from build123d import *

# Parameters (mm, degrees)
SKETCH2_W           = 1250
SKETCH2_H           = 250
BOSS_EXTRUDE1_DEPTH = 10
SKETCH3_W           = 25
SKETCH3_H           = 250
BOSS_EXTRUDE2_DEPTH = 300
SKETCH4_W           = 15
SKETCH4_H           = 10
BOSS_EXTRUDE3_DEPTH = 1200
FILLET1_R           = 5
FILLET3_R           = 5


with BuildPart() as part:
    # Sketch2 → Boss-Extrude1 (new body)
    with BuildSketch(Plane(origin=(0, 0, 0), x_dir=(1, 0, 0), z_dir=(0, 1, 0))):
        with Locations((546.563322885, -102.85317352)):
            Rectangle(SKETCH2_W, SKETCH2_H)
    extrude(amount=BOSS_EXTRUDE1_DEPTH)

    # Sketch3 → Boss-Extrude2 (add)
    with BuildSketch(Plane(origin=(0, 10, 0), x_dir=(1, 0, 0), z_dir=(0, 1, 0))):
        with Locations((-65.936677115, -102.85317352)):
            Rectangle(SKETCH3_W, SKETCH3_H)
        with Locations((1159.063322885, -102.85317352)):
            Rectangle(SKETCH3_W, SKETCH3_H)
    extrude(amount=BOSS_EXTRUDE2_DEPTH)

    # Sketch4 → Boss-Extrude3 (add)
    with BuildSketch(Plane(origin=(-53.436677115, 0, 0), x_dir=(0, 0, -1), z_dir=(1, 0, 0))):
        with Locations((-170.35317352, 175)):
            Rectangle(SKETCH4_W, SKETCH4_H)
        with Locations((-35.35317352, 175)):
            Rectangle(SKETCH4_W, SKETCH4_H)
    extrude(amount=BOSS_EXTRUDE3_DEPTH)

    # Fillet1
    fillet1_edges = [part.edges().sort_by_distance(p)[0] for p in [
        (546.563322885, 170, 177.85317352),
        (546.563322885, 170, 162.85317352),
    ]]
    fillet(fillet1_edges, radius=FILLET1_R)

    # Fillet3
    fillet3_edges = [part.edges().sort_by_distance(p)[0] for p in [
        (546.563322885, 170, 42.85317352),
        (546.563322885, 170, 27.85317352),
    ]]
    fillet(fillet3_edges, radius=FILLET3_R)


solid = part.part
The model under review builds one solid part; all positions refer to its coordinate system, in mm. Coordinates: 2 decimals unless noted, no trailing zeros. Loops run counter-clockwise (first coordinate to the right, second up) from the corner with the lowest first, then second, coordinate; pieces in that order, holes last. Notation, with made-up numbers: (40.5, 53) -> (56.5, 53) arc R18 ccw to (56.5, 64) -> close; hole circle Ø4 at (-7.75, -21.5). An arc over 180 degrees is marked (long way). Use a Markdown table: item, result. Add a question column.
1. Add section A-A on y = 127. Write out the cut boundary in (x, z), plus the area to 3 significant figures.
2. Add section B-B on x = 958. Write out the cut boundary in (y, z).
3. To check wall thickness, follow line 1 (X direction, y = 225, z = 1.5); line 2 (Y direction, x = 672, z = 122). State the ranges of each line that lie inside material, in increasing order.
4. Clearance check with flat-ended pins moving along their axes: pin 1 Ø5.5 at (x, y) = (458.5, 178) entering from +Z; pin 2 Ø5 at (x, z) = (258, 171) entering from +Y; pin 3 Ø5.5 at (x, y) = (464, 178.5) entering from -Z. State where each tip first meets the part, or that it passes through.
5. Draft analysis for pull direction X (two halves, no side actions). For faces 1 (the face through (538, 10, 101)), 2 (the face through (-66, 310, 101)), 3 (the face through (1171.563, 153, 105)), 4 (the face through (-78.437, 153, 105)), state which applies: pulls with the +X half, pulls with the -X half, needs draft (parallel to the pull), parting line crosses it, or undercut.
6. Add section C-C on z = 208. Write out the cut boundary in (x, y).
Returned:
| question | item | result |
|---|---|---|
| 1 | outline | (-78.44, -22.15) -> (-53.44, -22.15) -> (-53.44, 227.85) -> (-78.44, 227.85) -> close; (1146.56, -22.15) -> (1171.56, -22.15) -> (1171.56, 227.85) -> (1146.56, 227.85) -> close |
| 1 | area | 12,500 mm² |
| 2 | outline | (0, -22.15) -> (10, -22.15) -> (10, 227.85) -> (0, 227.85) -> close; (170, 32.85) arc R5 ccw to (175, 27.85) -> (180, 27.85) -> (180, 42.85) -> (175, 42.85) arc R5 ccw to (170, 37.85) -> close; (170, 167.85) arc R5 ccw to (175, 162.85) -> (180, 162.85) -> (180, 177.85) -> (175, 177.85) arc R5 ccw to (170, 172.85) -> close |
| 3 | line 1 | x = -78.44 to -53.44, 1146.56 to 1171.56 |
| 3 | line 2 | y = 0 to 10 |
| 4 | pin 1 | stops at z = 177.85 |
| 4 | pin 2 | stops at y = 180 |
| 4 | pin 3 | stops at z = 27.85 |
| 5 | face 1 | undercut |
| 5 | face 2 | needs draft |
| 5 | face 3 | pulls with the +X half |
| 5 | face 4 | pulls with the -X half |
| 6 | outline | (-78.44, 0) -> (1171.56, 0) -> (1171.56, 310) -> (1146.56, 310) -> (1146.56, 10) -> (-53.44, 10) -> (-53.44, 310) -> (-78.44, 310) -> close |
